Autodesk Inventor part; units mm, degrees
ref_plane "YZ Plane" through (0, 0, 0) normal (1, 0, 0) x (0, 1, 0)
ref_plane "XZ Plane" through (0, 0, 0) normal (0, 1, 0) x (-1, 0, 0)
ref_plane "XY Plane" through (0, 0, 0) normal (0, 0, 1) x (1, 0, 0)
sketch "Sketch1" plane through (0, 0, 0) normal (0, 0, 1) x (1, 0, 0)
  line L0 (0, 0) -> (0, 29.21)
  line L1 (0, 29.21) -> (-12.7, 29.21)
  line L2 (-12.7, 29.21) -> (-12.7, 22.86)
  line L3 (-12.7, 22.86) -> (-6.35, 22.86)
  line L4 (-6.35, 22.86) -> (-6.35, 16.51)
  line L5 (-6.35, 16.51) -> (-3.175, 16.51)
  line L6 (-3.175, 16.51) -> (-3.175, 0)
  line L7 (-3.175, 0) -> (0, 0)
  dimension "d0" = 29.21
  dimension "d1" = 12.7
  dimension "d2" = 6.35
  dimension "d3" = 6.35
  dimension "d4" = 6.35
  dimension "d5" = 3.175
revolve "Revolution1" add sketch "Sketch1" angle 360 about axis through (0, 0, 0) along (0, 1, 0)
sketch "Sketch2" plane through (0, 29.21, 0) normal (0, 1, 0) x (1, 0, 0)
  circle A0 centre (0, 0) radius 9.906
  dimension "d7" = 19.812
sketch "Sketch3" plane through (0, 29.21, 0) normal (0, 1, 0) x (1, 0, 0)
  line L0 (0, 0) -> (-3.287, 12.2673)
  line L1 (0, 0) -> (0, 12.62)
  dimension "d8" = 12.7
  dimension "d9" = 15
hole "Hole1" at (-3.287, 29.21, -12.2673) direction (0, -1, 0) diameter 3.556 end through all
pattern_circular "Circular Pattern1" count 12 over 360 about axis through (0, 26.035, 0) along (0, 1, 0) of "Hole1"
hole "Hole2" at (0, 29.21, 0) direction (0, -1, 0) diameter 19.812 depth 1.27
thread "Thread1"
properties part number "Lopez_Knob" material "Polypropylene"
Part model, mm, in its own coordinate system. A direction names the side the tool comes from. Round coordinates to 2 decimals unless told otherwise and drop trailing zeros. Order: outer loops, then holes, each group sorted by start corner. A loop starts at its lowest first (then second) coordinate and runs counter-clockwise, first axis right, second up. Notation, with made-up numbers: (4.25, 45) -> (26.25, 45) arc R24 cw to (26.25, 68) -> close; hole circle Ø8 at (-5.75, 77). An arc over 180 degrees is marked (long way). Put each result on its own line as item: value.
Q1. Band-saw the part on D-D (z = 11). Give the cut face in (x, y), and give its area (3 significant figures).
From the geometry:
outline: (-6.35, 22.86) -> (-4.53, 22.86) -> (-4.53, 29.21) -> (-6.35, 29.21) -> close; (-2.04, 22.86) -> (2.04, 22.86) -> (2.04, 29.21) -> (-2.04, 29.21) -> close; (4.53, 22.86) -> (6.35, 22.86) -> (6.35, 29.21) -> (4.53, 29.21) -> close
area: 48.9 mm2
Q2. Pin check, flat tips, straight feed: pin 1 Ø3 at (x, z) = (-7, 4) entering from -Y; pin 2 Ø6 at (x, y) = (3.5, 21) entering from +Z; pin 3 Ø4 at (x, y) = (-10, 21) entering from +Z. Stop position of each tip, or through.
From the geometry:
pin 1: stops at y = 22.86
pin 2: stops at z = 12.65
pin 3: stops at z = 7.64
Q3. Band-saw the part on A-A (x = 0). Give the cut face in (y, z) (3 decimals).
From the geometry:
outline: (0, -3.175) -> (16.51, -3.175) -> (16.51, -6.35) -> (22.86, -6.35) -> (22.86, -12.7) -> (29.21, -12.7) -> (29.21, -9.906) -> (27.94, -9.906) -> (27.94, 9.906) -> (29.21, 9.906) -> (29.21, 12.7) -> (22.86, 12.7) -> (22.86, 6.35) -> (16.51, 6.35) -> (16.51, 3.175) -> (0, 3.175) -> close
Q4. Tool access for faces 5 (the face through (1.38, 19.64, 6.2)), 6 (the face through (7.75, 25.991, -7.697)): list every direction of +Z, -Z, +X, -X, +Y, -Y with a clear straight run to the whole face (end or side of a thin tool).
From the geometry:
face 5: -Y
face 6: +Y, -Y
Q5. Band-saw the part on B-B (y = 25.5). Give the cut face in (x, z), and give its area (3 significant figures).
From the geometry:
outline: (-12.61, -1.54) arc R1.78 cw to (-11.69, -4.97) arc R12.7 ccw to (-10.15, -7.64) arc R1.78 cw to (-7.64, -10.15) arc R12.7 ccw to (-4.97, -11.69) arc R1.78 cw to (-1.54, -12.61) arc R12.7 ccw to (1.54, -12.61) arc R1.78 cw to (4.97, -11.69) arc R12.7 ccw to (7.64, -10.15) arc R1.78 cw to (10.15, -7.64) arc R12.7 ccw to (11.69, -4.97) arc R1.78 cw to (12.61, -1.54) arc R12.7 ccw to (12.61, 1.54) arc R1.78 cw to (11.69, 4.97) arc R12.7 ccw to (10.15, 7.64) arc R1.78 cw to (7.64, 10.15) arc R12.7 ccw to (4.97, 11.69) arc R1.78 cw to (1.54, 12.61) arc R12.7 ccw to (-1.54, 12.61) arc R1.78 cw to (-4.97, 11.69) arc R12.7 ccw to (-7.64, 10.15) arc R1.78 cw to (-10.15, 7.64) arc R12.7 ccw to (-11.69, 4.97) arc R1.78 cw to (-12.61, 1.54) arc R12.7 ccw to start
area: 449 mm2
Q6. Pull direction Z, two halves, no side cores. Call faces 1 (the face through (10.56, 25.99, -2.79)), 2 (the face through (0, 0, 0)), 3 (the face through (-10.54, 25.99, -2.86)), 4 (the face through (0.69, 8.14, 3.1)): pulls with the +Z half, pulls with the -Z half, needs draft (parallel to the pull), parting line crosses it, or undercut.
From the geometry:
face 1: undercut
face 2: needs draft
face 3: undercut
face 4: parting line crosses it
Q7. Band-saw the part on C-C (z = -9.5). Give the cut face in (x, y).
From the geometry:
outline: (-7.28, 22.86) -> (7.28, 22.86) -> (7.28, 29.21) -> (2.81, 29.21) -> (2.81, 27.94) -> (-2.81, 27.94) -> (-2.81, 29.21) -> (-7.28, 29.21) -> close
Q8. Wall check: line 1 (X direction, y = 28.35, z = 0); line 2 (Y direction, x = 6.5, z = 2.25). Give the ranges that are in metal, low to high. Write a range as [from, to].
From the geometry:
line 1: x = [-12.7, -9.91], [9.91, 12.7]
line 2: y = [22.86, 27.94]
